```python
from build123d import *

# Parameters (mm, degrees)
F1_DEPTH = 30
F2_R     = 11
F3_DEPTH = 20
F5_D     = 4.4
F6_D     = 3.3


with BuildPart() as f1:
    # F0 (on Front) → F1 (new body, symmetric)
    with BuildSketch(Plane.XZ):
        Polygon((-8, 40), (-10, 40), (-10, 0), (0, 0), (10, 0), (10, 40), (8, 40), (8, 2), (0, 2), (-8, 2), align=None)
    extrude(amount=F1_DEPTH, both=True)

    # F2 (on face) → F3 (cut, through all)
    with BuildSketch(Plane(origin=(-10, 0, 0), x_dir=(0, -1, 0), z_dir=(-1, 0, 0))):
        with Locations((0, 21)):
            Circle(F2_R)
    extrude(amount=-F3_DEPTH, mode=Mode.SUBTRACT)

    # F5 (through all)
    with Locations(Plane.XY.offset(2)):
        with Locations((0, 25), (0, -25)):
            Hole(F5_D / 2)

    # F6 (through all)
    with Locations(Plane(origin=(-10, 0, 0), x_dir=(0, -1, 0), z_dir=(-1, 0, 0))):
        with Locations((-26, 36), (26, 36)):
            Hole(F6_D / 2)


solid = f1.part
```
CAD build for the part. Positions are in the model's coordinates, mm. A direction names the side the tool comes from. Coordinates: 2 decimals unless noted, no trailing zeros. Order: outer loops, then holes, each group sorted by start corner. A loop starts at its lowest first (then second) coordinate and runs counter-clockwise, first axis right, second up. Notation, with made-up numbers: M 83.25,42 L 135.25,42 A33 ccw 135.25,74 Z; hole C 40,-38.5 d2. An arc over 180 degrees is marked long. Write each question's results on one line, items separated by ' | '. Start each with the question number.
Q1. Cut at A-A (z = 5.5). List the corners of the cut face in (x, y).
Q2. Drill centre lines: probe 1 along Y at (x, z) = (0, 1.5); probe 2 along X at (y, z) = (15, 32); probe 3 along Z at (x, y) = (-8.75, 26). Where is each one in solid material? Low to high. Write a range as from..to.
Q3. Pull direction Z, two halves, no side cores. Call faces 1 (the flat face through (-8.2, 30, 17.1)), 2 (the flat face through (9, 0, 40)), 3 (the cylindrical face through (8.99, 2.38, 10.26)): +Z half, -Z half, draft (parallel to the pull), parting line (faces both ways), or undercut.
Q4. Flat gauge pin, fed straight in: P1, Ø6, axis at x = -4, y = -18, coming from the +Z side. Where does the tip first touch, or does it go through?
Q5. Which spindle directions (+Z, -Z, +X, -X, +Y, -Y) get a long thin tool onto all of the face, cutting with end or side? Do faces 4 (the cylindrical face through (-8.986, -27.216, 37.115)), 5 (the flat face through (0, 0, 2)). Say none if no direction does.
Q6. Cut at D-D (x = 0). List the corners of the cut face in (y, z), then the cut area to 3 significant figures.
Q7. Cut at B-B (z = 21). List the corners of the cut face in (x, y).
Q8. Cut at C-C (y = 0). List the corners of the cut face in (x, z).
Found:
1) outline: M -10,-30 L -8,-30 L -8,30 L -10,30 Z; M 8,-30 L 10,-30 L 10,30 L 8,30 Z
2) probe 1: -30..-27.2, -22.8..22.8, 27.2..30 | probe 2: -10..-8, 8..10 | probe 3: 0..34.35, 37.65..40
3) face 1: draft | face 2: +Z half | face 3: undercut
4) P1: z = 2
5) face 4: +X, -X | face 5: +Z, +Y, -Y
6) outline: M -30,0 L -27.2,0 L -27.2,2 L -30,2 Z; M -22.8,0 L 22.8,0 L 22.8,2 L -22.8,2 Z; M 27.2,0 L 30,0 L 30,2 L 27.2,2 Z | area: 102 mm²
7) outline: M -10,-30 L -8,-30 L -8,-11 L -10,-11 Z; M -10,11 L -8,11 L -8,30 L -10,30 Z; M 8,-30 L 10,-30 L 10,-11 L 8,-11 Z; M 8,11 L 10,11 L 10,30 L 8,30 Z
8) outline: M -10,0 L 10,0 L 10,10 L 8,10 L 8,2 L -8,2 L -8,10 L -10,10 Z; M -10,32 L -8,32 L -8,40 L -10,40 Z; M 8,32 L 10,32 L 10,40 L 8,40 Z
